from build123d import *

# Parameters (mm, degrees)
F0_W     = 2000
F0_H     = 800
F1_DEPTH = 40


with BuildPart() as f1:
    # F0 (on Top) → F1 (new body)
    with BuildSketch(Plane.XY):
        Rectangle(F0_W, F0_H)
        with BuildLine():
            Line((850, -360), (-850, -360))
            Line((-850, -360), (-850, -112.5))
            ThreePointArc((-850, -112.5), (-912.5, -50), (-850, 12.5))
            Line((-850, 12.5), (-850, 360))
            Line((-850, 360), (850, 360))
            Line((850, 360), (850, 12.65))
            ThreePointArc((850, 12.65), (912.65, -50), (850, -112.65))
            Line((850, -112.65), (850, -360))
        make_face(mode=Mode.SUBTRACT)
    extrude(amount=F1_DEPTH)


solid = f1.part
Geometry check sheet. Reference: the model listing, model coordinates, mm. A direction names the side the tool comes from. Give positions to 0.01 mm unless a question says otherwise; leave off trailing zeros. Loops run counter-clockwise (first coordinate to the right, second up) from the corner with the lowest first, then second, coordinate; pieces in that order, holes last.
(1) Set-up check for faces 4 (the flat face through (-850, 184, 20)), 5 (the flat face through (-1000, -6, 20)): record each of +Z, -Z, +X, -X, +Y, -Y from which the full face is reachable in a straight line by a thin tool's end or side.
From the geometry:
face 4: +Z, -Z
face 5: +Z, -Z, -X, +Y, -Y
(2) Section check B-B on y = -297. Record the cut outline in (x, z), then the cut area to 3 significant figures.
From the geometry:
outline: (-1000, 0) - (-850, 0) - (-850, 40) - (-1000, 40) - close; (850, 0) - (1000, 0) - (1000, 40) - (850, 40) - close
area: 12,000 mm2
(3) Release check for a two-part mould opening along X. For faces 1 (the flat face through (-79, 387, 40)), 2 (the cylindrical face through (-912.485, -51.374, 19.72)), 3 (the flat face through (1000, -6, 20)) record: released by +X, released by -X, zero draft, split by the parting line, or undercut.
From the geometry:
face 1: zero draft
face 2: undercut
face 3: released by +X
(4) Thickness scan on L1, parallel to Y at x = 281, z = 25; L2, parallel to X at y = 190.5, z = 5; L3, parallel to X at y = -95, z = 3. Record the ranges inside material, lowest first.
From the geometry:
L1: y = -400 to -360, 360 to 400
L2: x = -1000 to -850, 850 to 1000
L3: x = -1000 to -893.37, 893.59 to 1000
(5) Section check C-C on z = 17.5. Record the cut outline in (x, y), then the cut area to 3 significant figures.
From the geometry:
outline: (-1000, -400) - (1000, -400) - (1000, 400) - (-1000, 400) - close; hole (-850, -360) - (850, -360) - (850, -112.65) arc R62.65 ccw to (850, 12.65) - (850, 360) - (-850, 360) - (-850, 12.5) arc R62.5 ccw to (-850, -112.5) - close
area: 364,000 mm2
(6) Section check A-A on x = -300.5. Record the cut outline in (y, z), then the cut area to 3 significant figures.
From the geometry:
outline: (-400, 0) - (-360, 0) - (-360, 40) - (-400, 40) - close; (360, 0) - (400, 0) - (400, 40) - (360, 40) - close
area: 3,200 mm2
